Could you check a few things on this model? Use its own coordinates, in mm. A direction names the side the tool comes from. Coordinates: 2 decimals unless noted, no trailing zeros. Loops run counter-clockwise (first coordinate to the right, second up) from the corner with the lowest first, then second, coordinate; pieces in that order, holes last. Notation, with made-up numbers: (55.5, 37) -> (84.5, 37) arc R21 ccw to (84.5, 64) -> close; hole circle Ø8 at (67.25, 61.5). An arc over 180 degrees is marked (long way). One line per question, with ' | ' between items. Start each with the question number.
(1) If I drill on line 1 along Z through (x, y) = (553.5, 6); line 2 along X through (y, z) = (4.75, -50); line 3 along Z through (x, y) = (553.5, 9), over which ranges is the centre line in solid material (lowest first)?
(2) Which directions (+Z, -Z, +X, -X, +Y, -Y) give clear straight access to the entire face, cutting with the end or side of a thin tool? Please do faces 1 (the face through (33.804, 3.451, -60.492)), 2 (the face through (288, 7, -100)).
(3) Suppose I cut it at A-A (y = 2.5). Please give me the cut outline in (x, z), plus the area to 3 significant figures.
(4) Suppose I cut it at B-B (z = -50). Please give me the cut outline in (x, y).
(5) I'm going to push flat-ended pins straight in: pin 1 Ø6.5 at (x, z) = (31.5, -17) entering from +Y; pin 2 Ø20 at (x, z) = (30.5, -50) entering from -Y. Where does each tip first touch, or does it pass through?
```python
from build123d import *

# Parameters (mm, degrees)
CROQUIS1_W              = 585
CROQUIS1_H              = 100
CROQUIS1_R              = 4
SALIENTE_EXTRUIR1_DEPTH = 15
CROQUIS2_R              = 11
CORTAR_EXTRUIR1_DEPTH   = 7


with BuildPart() as part:
    # Croquis1 → Saliente-Extruir1 (new body)
    with BuildSketch(Plane(origin=(0, 0, 0), x_dir=(1, 0, 0), z_dir=(0, 1, 0))):
        with Locations((292.5, 50)):
            Rectangle(CROQUIS1_W, CROQUIS1_H)
        with Locations(Location((31.5, 83, 0), (0, 0, 270))):
            Circle(CROQUIS1_R, mode=Mode.SUBTRACT)
        with Locations(Location((31.5, 17, 0), (0, 0, 270))):
            Circle(CROQUIS1_R, mode=Mode.SUBTRACT)
        with Locations(Location((553.5, 17, 0), (0, 0, 90))):
            Circle(CROQUIS1_R, mode=Mode.SUBTRACT)
        with Locations(Location((553.5, 83, 0), (0, 0, 90))):
            Circle(CROQUIS1_R, mode=Mode.SUBTRACT)
    extrude(amount=SALIENTE_EXTRUIR1_DEPTH)

    # Croquis2 → Cortar-Extruir1 (cut)
    with BuildSketch(Plane.XZ):
        with Locations(Location((30.5, -50, 0), (0, 0, 270))):
            Circle(CROQUIS2_R)
        with Locations(Location((554.5, -50, 0), (0, 0, 90))):
            Circle(CROQUIS2_R)
    extrude(amount=-CORTAR_EXTRUIR1_DEPTH, mode=Mode.SUBTRACT)


solid = part.part
```
Checks:
1) line 1: z = -100 to -87, -79 to -60.95, -39.05 to -21, -13 to 0 | line 2: x = 0 to 19.5, 41.5 to 543.5, 565.5 to 585 | line 3: z = -100 to -87, -79 to -21, -13 to 0
2) face 1: -Y | face 2: -Z, +X, -X, +Y, -Y
3) outline: (0, -100) -> (585, -100) -> (585, 0) -> (0, 0) -> close; hole circle Ø22 at (30.5, -50); hole circle Ø8 at (31.5, -83); hole circle Ø8 at (31.5, -17); hole circle Ø22 at (554.5, -50); hole circle Ø8 at (553.5, -83); hole circle Ø8 at (553.5, -17) | area: 57,500 mm^2
4) outline: (0, 0) -> (19.5, 0) -> (19.5, 7) -> (41.5, 7) -> (41.5, 0) -> (543.5, 0) -> (543.5, 7) -> (565.5, 7) -> (565.5, 0) -> (585, 0) -> (585, 15) -> (0, 15) -> close
5) pin 1: passes through | pin 2: stops at y = 7
